Input: part model. Units: mm. Frame: model coordinates. A direction names the side the tool comes from. Give positions to 0.01 mm unless a question says otherwise; leave off trailing zeros. Loops run counter-clockwise (first coordinate to the right, second up) from the corner with the lowest first, then second, coordinate; pieces in that order, holes last. Notation, with made-up numbers: M 76.5,72 L 112.5,72 A8 ccw 112.5,81 Z; hole C 84.5,50.25 d10. An arc over 180 degrees is marked long. Use a Markdown table: item, result. Add a question column.
from build123d import *

# Parameters (mm, degrees)
BOSS_EXTRUDE1_DEPTH                                = 25.4
FILLET1_R                                          = 127
FILLET2_R                                          = 25.4
WHEEL_SLOT_DEPTH                                   = 25.4
PEDAL_SLOT_DEPTH                                   = 25.4
CSK_FOR_10_FLAT_HEAD_MACHINE_SCREW_100_D           = 5.1054
CSK_FOR_10_FLAT_HEAD_MACHINE_SCREW_100_CSINK_D     = 9.779
CSK_FOR_10_FLAT_HEAD_MACHINE_SCREW_100_CSINK_ANGLE = 100


# Read off the part's stored shape, not the designer's step: wheel slot, pedal slot
with BuildPart() as part:
    # Sketch1 → Boss-Extrude1 (new body)
    with BuildSketch(Plane.XY):
        Polygon((0, 0), (-193.132194655, 334.514773719), (-19.646968374, 635), (107.353031626, 635), (-11.089113546, 889), (-576.905448196, 889), (-897.037642851, 334.514773719), (-703.905448196, 0), align=None)
    extrude(amount=BOSS_EXTRUDE1_DEPTH)

    # Fillet1
    fillet1_edges = [part.edges().sort_by_distance(p)[0] for p in [
        (-897.037642851, 334.514773719, 12.7),
        (-193.132194655, 334.514773719, 12.7),
    ]]
    fillet(fillet1_edges, radius=FILLET1_R)

    # Fillet2
    fillet2_edges = [part.edges().sort_by_distance(p)[0] for p in [
        (-576.905448196, 889, 12.7),
        (-11.089113546, 889, 12.7),
        (107.353031626, 635, 12.7),
        (-19.646968374, 635, 12.7),
    ]]
    fillet(fillet2_edges, radius=FILLET2_R)

    # wheel slot outline → wheel slot (cut)
    with BuildSketch(Plane.XY):
        with BuildLine():
            Line((-154.207271537, 714.375), (-154.207271537, 809.625))
            ThreePointArc((-154.207271537, 809.625), (-157.382271537, 812.8), (-160.557271537, 809.625))
            Line((-160.557271537, 809.625), (-160.557271537, 714.375))
            ThreePointArc((-160.557271537, 714.375), (-157.382271537, 711.2), (-154.207271537, 714.375))
        make_face()
        with BuildLine():
            Line((-27.207271537, 714.375), (-27.207271537, 809.625))
            ThreePointArc((-27.207271537, 809.625), (-30.382271537, 812.8), (-33.557271537, 809.625))
            Line((-33.557271537, 809.625), (-33.557271537, 714.375))
            ThreePointArc((-33.557271537, 714.375), (-30.382271537, 711.2), (-27.207271537, 714.375))
        make_face()
    extrude(amount=WHEEL_SLOT_DEPTH, mode=Mode.SUBTRACT)

    # pedal slot outline → pedal slot (cut)
    with BuildSketch(Plane.XY):
        with BuildLine():
            Line((-720.725, 352.425), (-295.275, 352.425))
            ThreePointArc((-295.275, 352.425), (-292.1, 355.6), (-295.275, 358.775))
            Line((-295.275, 358.775), (-720.725, 358.775))
            ThreePointArc((-720.725, 358.775), (-723.9, 355.6), (-720.725, 352.425))
        make_face()
        with BuildLine():
            Line((-688.030448196, 260.789543073), (-262.580448196, 260.789543073))
            ThreePointArc((-262.580448196, 260.789543073), (-259.405448196, 263.964543073), (-262.580448196, 267.139543073))
            Line((-262.580448196, 267.139543073), (-688.030448196, 267.139543073))
            ThreePointArc((-688.030448196, 267.139543073), (-691.205448196, 263.964543073), (-688.030448196, 260.789543073))
        make_face()
        with BuildLine():
            Line((-637.230448196, 172.801362049), (-211.780448196, 172.801362049))
            ThreePointArc((-211.780448196, 172.801362049), (-208.605448196, 175.976362049), (-211.780448196, 179.151362049))
            Line((-211.780448196, 179.151362049), (-637.230448196, 179.151362049))
            ThreePointArc((-637.230448196, 179.151362049), (-640.405448196, 175.976362049), (-637.230448196, 172.801362049))
        make_face()
    extrude(amount=PEDAL_SLOT_DEPTH, mode=Mode.SUBTRACT)

    # CSK for #10 Flat Head Machine Screw (100)1 (through all)
    with Locations(Plane.XY.offset(25.4)):
        with Locations((-530.490751359, 876.3), (-530.490751359, 825.5), (-498.740751359, 876.3), (-447.940751359, 876.3), (-397.140751359, 876.3), (-346.340751359, 876.3), (-295.540751359, 876.3), (-244.740751359, 876.3), (-530.490751359, 774.7), (-530.490751359, 723.9), (-530.490751359, 673.1), (-530.490751359, 622.3), (-530.490751359, 571.5), (-193.940751359, 876.3)):
            CounterSinkHole(CSK_FOR_10_FLAT_HEAD_MACHINE_SCREW_100_D / 2, CSK_FOR_10_FLAT_HEAD_MACHINE_SCREW_100_CSINK_D / 2, counter_sink_angle=CSK_FOR_10_FLAT_HEAD_MACHINE_SCREW_100_CSINK_ANGLE)


solid = part.part
1) Contact query for flat-ended pins moving along their axis: P1, Ø12.5, axis at y = 778, z = 6.5, coming from the +X side; P2, Ø4, axis at x = -447.94, y = 876.3, coming from the +Z side; P3, Ø12.5, axis at x = -434.5, z = 16, coming from the -Y side; P4, Ø7.5, axis at y = 743.5, z = 15, coming from the -X side (3 decimals). Output: stop coordinate, or through.
2) Pull-direction query (X, two-part tool) for faces 4 (the flat face through (-422, 179.151, 13)), 5 (the cylindrical face through (-13.45, 884.91, 12.88)), 6 (the cylindrical face through (-877.387, 335.446, 12.878)), 7 (the flat face through (-27.207, 761, 13)); classes: pulls with the +X half, pulls with the -X half, needs draft (parallel to the pull), parting line crosses it, or undercut.
3) Section query A-A, the plane x = -657. Return the cut outline in (y, z) (3 decimals).
4) Reachability of faces 1 (the flat face through (-77.14, 133.61, 12.52)), 2 (the flat face through (-33.557, 763, 13)), 3 (the flat face through (-783.236, 137.404, 12.522)) from +Z, -Z, +X, -X, +Y, -Y: full face, straight path, thin tool, end or side. Return the list, or none.
5) Ray query, line 1 (Y direction, x = -342, z = 6.25) (3 decimals); line 2 (Y direction, x = -275.5, z = 17.5); line 3 (X direction, y = 785, z = 1.75). Return the intervals inside material, ascending. Write a range as [from, to].
6) Section query B-B, the plane z = 8.75. State how many separate pieces and enclosed holes the cut face has, and give its area (3 significant figures).
Entries:
| question | item | result |
|---|---|---|
| 1 | P1 | stops at x = 43.59 |
| 1 | P2 | passes through |
| 1 | P3 | stops at y = 0 |
| 1 | P4 | stops at x = -663.075 |
| 2 | face 4 | undercut |
| 2 | face 5 | pulls with the +X half |
| 2 | face 6 | pulls with the -X half |
| 2 | face 7 | undercut |
| 3 | outline | M 0,0 L 260.79,0 L 260.79,25.4 L 0,25.4 Z; M 267.14,0 L 352.425,0 L 352.425,25.4 L 267.14,25.4 Z; M 358.775,0 L 750.272,0 L 750.272,25.4 L 358.775,25.4 Z |
| 4 | face 1 | +Z, -Z, +X |
| 4 | face 2 | +Z, -Z |
| 4 | face 3 | +Z, -Z, -X, -Y |
| 5 | line 1 | y = [0, 172.801], [179.151, 260.79], [267.14, 352.425], [358.775, 889] |
| 5 | line 2 | y = [0, 172.8], [179.15, 260.79], [267.14, 889] |
| 5 | line 3 | x = [-636.95, -160.56], [-154.21, -33.56], [-27.21, 37.41] |
| 6 | separate pieces | 1 |
| 6 | enclosed holes | 19 |
| 6 | area | 614,000 mm² |
